Here's how the part is built. I have some questions about the finished solid (model axes, mm). Face numbers are marked on the shaded views. A direction names the side the tool comes from. Give positions to 0.01 mm unless a question says otherwise; leave off trailing zeros. Loops run counter-clockwise (first coordinate to the right, second up) from the corner with the lowest first, then second, coordinate; pieces in that order, holes last. Notation, with made-up numbers: M 66,15.25 L 124,15.25 A11 cw 124,26.25 Z; hole C 16,61 d9. An arc over 180 degrees is marked long. Answer as CSV lines item,"result". Start each with the question number.
Item 1: I want a section at A-A on x = -3.75. List the corners of the cut face in (y, z) for me.
Item 2: I want a section at C-C on z = -11. List the corners of the cut face in (x, y) for me.
Item 3: Will these pins go through, and if not, where does the flat tip stop? P1, Ø5, axis at x = 7, y = -6, coming from the -Z side; P2, Ø1.9, axis at x = -5.5, z = -35, coming from the -Y side; P3, Ø8.5, axis at y = 0.5, z = -29.5, coming from the +X side; P4, Ø3, axis at y = 6, z = 25.5, coming from the +X side.
Item 4: If I drill on line 1 along Z through (x, y) = (5.25, 0); line 2 along Y through (x, z) = (-4.75, 24.5); line 3 along X through (y, z) = (-2.5, -34), over which ranges is the centre line in solid material (lowest first)? Write a range as from..to.
Item 5: For the marked faces 1, 2 and 3, which set-ups out of +Z, -Z, +X, -X, +Y, -Y let a thin tool reach every point of the face, with its end or its side?
Item 6: I want a section at D-D on y = -7. List the corners of the cut face in (x, z) for me.
Autodesk Inventor part; units mm, degrees
ref_plane "YZ Plane" through (0, 0, 0) normal (1, 0, 0) x (0, 1, 0)
ref_plane "XZ Plane" through (0, 0, 0) normal (0, 1, 0) x (-1, 0, 0)
ref_plane "XY Plane" through (0, 0, 0) normal (0, 0, 1) x (1, 0, 0)
sketch "Sketch1" plane through (0, 0, 0) normal (1, 0, 0) x (0, 1, 0)
  circle A0 centre (0, 0) radius 4.572
  circle A1 centre (0, 0) radius 8.382
  dimension "d0" = 9.144
  dimension "d1" = 3.81
extrude "Extrusion1" add sketch "Sketch1" along normal blind 19.812
sketch "Sketch2" plane through (0, 0, 0) normal (-1, 0, 0) x (0, 0, 1)
  circle A0 centre (0, 0) radius 8.382
  circle A1 centre (0, 0) radius 7.747
  circle A2 centre (0, 0) radius 8.382
  dimension "d42" = 0
extrude "Extrusion2" add sketch "Sketch2" along normal blind 2.54 contours A0 | A1
sketch "Sketch10" plane through (0, 0, 0) normal (1, 0, 0) x (0, 0, -1)
  circle A0 centre (0, 0) radius 1.4542
  line L0 (-4.572, 1.4542) -> (4.572, 1.4542)
  line L1 (4.572, 1.4542) -> (4.572, -1.4542)
  line L2 (4.572, -1.4542) -> (-4.572, -1.4542)
  line L3 (-4.572, -1.4542) -> (-4.572, 1.4542)
  circle A1 centre (0, 0) radius 4.572
  dimension "d43" = 0
  dimension "d44" = 0
extrude "Extrusion7" cut sketch "Sketch10" against normal blind 22.225 contours A0 | A0 L0 A1 L2 | A0 L2 A1 L0 | A1 L3 L0 | L0 L1 A1 | A1 L1 L2 | L2 L3 A1
sketch "Sketch24" plane through (-2.54, 0, 0) normal (-1, 0, 0) x (0, 0, 1)
  line L0 (50.8, -3.81) -> (-50.8, -3.81)
  line L1 (-50.8, -3.81) -> (-50.8, 3.81)
  line L2 (-50.8, 3.81) -> (50.8, 3.81)
  line L3 (50.8, 3.81) -> (50.8, -3.81)
  line L4 (4.572, 1.4542) -> (4.572, -1.4542)
  line L5 (4.572, -1.4542) -> (-4.572, -1.4542)
  line L6 (-4.572, -1.4542) -> (-4.572, 1.4542)
  line L7 (-4.572, 1.4542) -> (4.572, 1.4542)
  circle A0 centre (0, 0) radius 8.382
  dimension "d90" = 101.6
  dimension "d91" = 50.8
  dimension "d92" = 3.81
  dimension "d93" = 3.81
extrude "Extrusion18" add sketch "Sketch24" along normal blind 6.35 contours L0 A0 L2 L3 | L0 A0 L2 | L0 L1 L2 A0
sketch "Sketch25" plane through (-2.54, 0, 0) normal (-1, 0, 0) x (0, 0, 1)
  line L0 (-7.466, 3.81) -> (7.466, 3.81)
  arc A0 (7.466, 3.81) -> (-7.466, 3.81) centre (0, 0) ccw
  line L1 (7.466, -3.81) -> (-7.466, -3.81)
  arc A1 (-7.466, -3.81) -> (7.466, -3.81) centre (0, 0) ccw
extrude "Extrusion19" add sketch "Sketch25" along normal blind 6.35
sketch "Sketch26" plane through (-2.54, -3.81, 7.466) normal (0, -1, 0) x (1, 0, 0)
  line L0 (0, 0) -> (0, 43.334)
  line L1 (0, 43.334) -> (-3.175, 43.334)
  line L2 (-3.175, 43.334) -> (-3.175, 36.984)
  line L3 (-3.175, 36.984) -> (0, 36.984)
  line L4 (0, 36.984) -> (0, 43.334)
  point P0 (2.54, -7.466)
  dimension "d98" = 3.175
  dimension "d99" = 6.35
extrude "Extrusion20" cut sketch "Sketch26" against normal blind 25.4
properties part number "LiftMotorHousingOne"
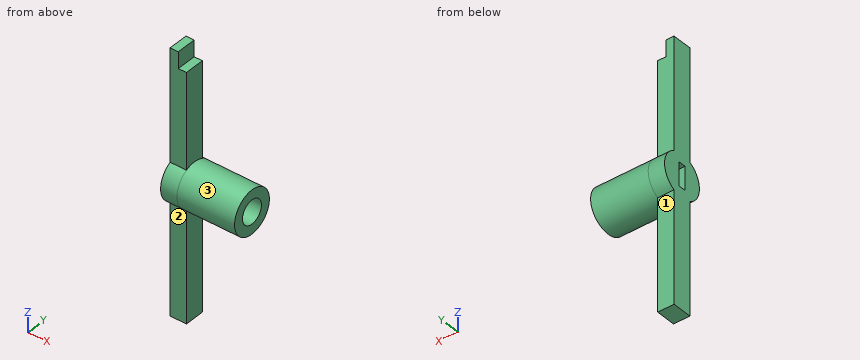
Result:
1,outline,"M -3.81,-50.8 L 3.81,-50.8 L 3.81,-7.47 A8.38 ccw 3.81,7.47 L 3.81,44.45 L -3.81,44.45 L -3.81,7.47 A8.38 ccw -3.81,-7.47 Z; hole M -1.45,-4.57 L 1.45,-4.57 L 1.45,4.57 L -1.45,4.57 Z"
2,outline,"M -8.89,-3.81 L -2.54,-3.81 L -2.54,3.81 L -8.89,3.81 Z"
3,P1,"z = -7.62"
3,P2,"y = -3.81"
3,P3,"x = -2.54"
3,P4,"through"
4,line 1,"-8.38..-4.57, 4.57..8.38"
4,line 2,"-3.81..3.81"
4,line 3,"-8.89..-2.54"
5,face 1,"-Z, +X, -X, +Y"
5,face 2,"-Z, +X, -X, -Y"
5,face 3,"+X"
6,outline,"M -8.89,-4.61 L 19.81,-4.61 L 19.81,4.61 L -8.89,4.61 Z"
